Here's how the part is built. I have some questions about the finished solid (model axes, mm). Face numbers are marked on the shaded views. A direction names the side the tool comes from. Coordinates: 2 decimals unless noted, no trailing zeros. Order: outer loops, then holes, each group sorted by start corner. A loop starts at its lowest first (then second) coordinate and runs counter-clockwise, first axis right, second up. Notation, with made-up numbers: (-1.75, -1) - (21.25, -1) arc R24 ccw to (21.25, 10) - close; hole circle Ø4 at (-33, -26.75). An arc over 180 degrees is marked (long way). Answer in a Markdown table with one row per item. Add a question column.
Item 1: I want a section at A-A (z = -13). Please give me the cut outline in (x, y), plus the area to 3 significant figures.
Item 2: I want a section at C-C (z = -25.5). Please give me the cut outline in (x, y), plus the area to 3 significant figures.
Item 3: If I drill on line 1 along Z through (x, y) = (-18, 17.5); line 2 along Z through (x, y) = (24, 2.25); line 3 along X through (y, z) = (13.5, 0), over which ranges is the centre line in solid material (lowest first)? Write a range as from..to.
Item 4: I want a section at B-B (y = 3.25). Please give me the cut outline in (x, z).
Item 5: Will these pins go through, and if not, where does the flat tip stop? pin 1 Ø1.8 at (x, y) = (21.5, 17) entering from +Z; pin 2 Ø6 at (y, z) = (14, -18.5) entering from -X; pin 3 Ø3 at (x, z) = (21, -7.5) entering from +Y.
Item 6: On a 3-axis mill with a long thin cutter (end or side, diameter ignored), from which of +Z, -Z, +X, -X, +Y, -Y can I reach the whole of each face in a straight line? I mean the marked faces 4, 5, 6 and 7. Say none if no direction works.
Item 7: Thinking about a two-plate mould opening in Z: for the marked faces 1, 2 and 3, which applies, +Z half, -Z half, draft (parallel to the pull), parting line (faces both ways), or undercut?
```python
from build123d import *

# Parameters (mm, degrees)
SKETCH1_W           = 45
SKETCH1_H           = 45
BOSS_EXTRUDE1_DEPTH = 25
SKETCH2_W           = 44
SKETCH2_H           = 24
BOSS_EXTRUDE2_DEPTH = 6
SKETCH3_R           = 2.5
BOSS_EXTRUDE3_DEPTH = 10.6
FILLET12_R          = 1
FILLET13_R          = 1
SKETCH4_W           = 5
SKETCH4_H           = 10.5
CUT_EXTRUDE1_DEPTH  = 10.5
SKETCH5_W           = 15
SKETCH5_H           = 10.5
BOSS_EXTRUDE4_DEPTH = 0.5
FILLET14_R          = 0.1


with BuildPart() as part:
    # Sketch1 → Boss-Extrude1 (new body)
    with BuildSketch(Plane(origin=(0, 0, 0), x_dir=(1, 0, 0), z_dir=(0, 1, 0))):
        with Locations((-3.078947368, 6.710526316)):
            Rectangle(SKETCH1_W, SKETCH1_H)
    extrude(amount=BOSS_EXTRUDE1_DEPTH)

    # Sketch2 → Boss-Extrude2 (add)
    with BuildSketch(Plane(origin=(19.421052632, 0, 0), x_dir=(0, 0, -1), z_dir=(1, 0, 0))):
        with Locations((6.710526316, 12.5)):
            Rectangle(SKETCH2_W, SKETCH2_H)
    extrude(amount=BOSS_EXTRUDE2_DEPTH)

    # Sketch3 → Boss-Extrude3 (add)
    with BuildSketch(Plane(origin=(25.421052632, 0, 0), x_dir=(0, 0, -1), z_dir=(1, 0, 0))):
        with Locations((18.710526316, 12.5)):
            Circle(SKETCH3_R)
        with Locations((-5.289473684, 12.5)):
            Circle(SKETCH3_R)
    extrude(amount=BOSS_EXTRUDE3_DEPTH)

    # Fillet12
    fillet12_edges = [part.edges().sort_by_distance(p)[0] for p in [
        (36.021052632, 12.5, 7.789473684),
    ]]
    fillet(fillet12_edges, radius=FILLET12_R)

    # Fillet13
    fillet13_edges = [part.edges().sort_by_distance(p)[0] for p in [
        (36.021052632, 12.5, -16.210526316),
    ]]
    fillet(fillet13_edges, radius=FILLET13_R)

    # Sketch4 → Cut-Extrude1 (cut)
    with BuildSketch(Plane.ZY.offset(25.578947368)):
        with Locations((-21.710526316, 13.203091604)):
            Rectangle(SKETCH4_W, SKETCH4_H)
        with Locations((-11.710526316, 13.203091604)):
            Rectangle(SKETCH4_W, SKETCH4_H)
    extrude(amount=-CUT_EXTRUDE1_DEPTH, mode=Mode.SUBTRACT)

    # Sketch5 → Boss-Extrude4 (add)
    with BuildSketch(Plane.ZY.offset(25.578947368)):
        with Locations((3.289473684, 13.203091604)):
            Rectangle(SKETCH5_W, SKETCH5_H)
    extrude(amount=BOSS_EXTRUDE4_DEPTH)

    # Fillet14
    fillet14_edges = [part.edges().sort_by_distance(p)[0] for p in [
        (-26.078947368, 13.203091604, -4.210526316),
        (-26.078947368, 7.953091604, 3.289473684),
        (-26.078947368, 13.203091604, 10.789473684),
        (-26.078947368, 18.453091604, 3.289473684),
    ]]
    fillet(fillet14_edges, radius=FILLET14_R)


solid = part.part
```
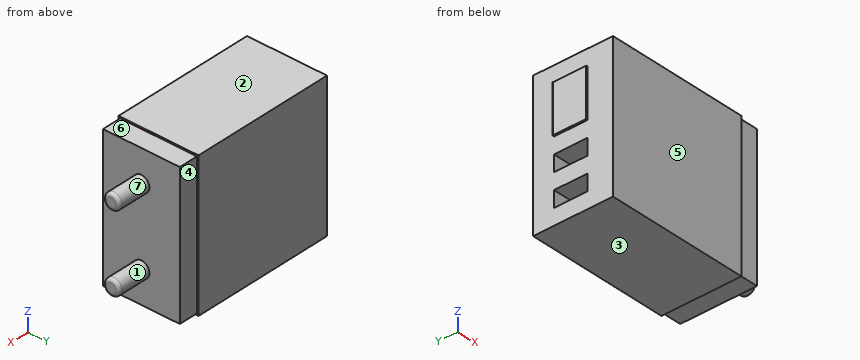
Values follow:
| question | item | result |
|---|---|---|
| 1 | outline | (-25.58, 0) - (19.42, 0) - (19.42, 0.5) - (25.42, 0.5) - (25.42, 24.5) - (19.42, 24.5) - (19.42, 25) - (-25.58, 25) - (-25.58, 18.45) - (-15.08, 18.45) - (-15.08, 7.95) - (-25.58, 7.95) - close |
| 1 | area | 1,160 mm^2 |
| 2 | outline | (-25.58, 0) - (19.42, 0) - (19.42, 0.5) - (25.42, 0.5) - (25.42, 24.5) - (19.42, 24.5) - (19.42, 25) - (-25.58, 25) - close |
| 2 | area | 1,270 mm^2 |
| 3 | line 1 | z = -29.21..-24.21, -19.21..-14.21, -9.21..15.79 |
| 3 | line 2 | z = -28.71..15.29 |
| 3 | line 3 | x = -26.08..25.42 |
| 4 | outline | (-25.58, -29.21) - (19.42, -29.21) - (19.42, -28.71) - (25.42, -28.71) - (25.42, 15.29) - (19.42, 15.29) - (19.42, 15.79) - (-25.58, 15.79) - close |
| 5 | pin 1 | stops at z = 15.29 |
| 5 | pin 2 | stops at x = -25.58 |
| 5 | pin 3 | stops at y = 24.5 |
| 6 | face 4 | +Z, -Z, +X, +Y |
| 6 | face 5 | +Z, -Z, +X, -X, -Y |
| 6 | face 6 | +Z, +X, +Y, -Y |
| 6 | face 7 | +X |
| 7 | face 1 | undercut |
| 7 | face 2 | +Z half |
| 7 | face 3 | -Z half |
